from build123d import *

# Parameters (mm, degrees)
SKETCH1_R           = 22.225
SKETCH1_R_2         = 8.001
BOSS_EXTRUDE1_DEPTH = 31.75
SKETCH2_R           = 1.5875
SKETCH2_R_2         = 8.001
CUT_EXTRUDE1_DEPTH  = 9.921875
FILLET1_R           = 3.175
SKETCH3_R           = 1.5875
CUT_EXTRUDE2_DEPTH  = 45.676210112


with BuildPart() as part:
    # Sketch1 → Boss-Extrude1 (new body)
    with BuildSketch(Plane(origin=(0, 0, 0), x_dir=(1, 0, 0), z_dir=(0, 1, 0))):
        with Locations(Location((0, 0, 0), (0, 0, 270))):
            Circle(SKETCH1_R)
        with Locations(Location((0, 0, 0), (0, 0, 270))):
            Circle(SKETCH1_R_2, mode=Mode.SUBTRACT)
    extrude(amount=BOSS_EXTRUDE1_DEPTH)

    # Sketch2 → Cut-Extrude1 (cut)
    # profile 1 of 31: a face of its own
    with BuildSketch(Plane.XZ):
        with BuildLine():
            ThreePointArc((-12.2555, 0), (-12.468184671, 0.79375), (-13.04925, 1.374815329))
            Line((-13.04925, 1.374815329), (-13.843, 0))
            Line((-13.843, 0), (-13.04925, -1.374815329))
            ThreePointArc((-13.04925, -1.374815329), (-12.468184671, -0.79375), (-12.2555, 0))
        make_face()
    # profile 2 of 31: a face of its own
    with BuildSketch(Plane.XZ):
        with BuildLine():
            Line((-13.843, 0), (-13.04925, 1.374815329))
            ThreePointArc((-13.04925, 1.374815329), (-15.4305, 0), (-13.04925, -1.374815329))
            Line((-13.04925, -1.374815329), (-13.843, 0))
        make_face()
    # profile 3 of 31: a face of its own
    with BuildSketch(Plane.XZ):
        with BuildLine():
            ThreePointArc((-12.2555, 0), (-12.468184671, 0.79375), (-13.04925, 1.374815329))
            Line((-13.04925, 1.374815329), (-13.843, 0))
            Line((-13.843, 0), (-13.04925, -1.374815329))
            ThreePointArc((-13.04925, -1.374815329), (-12.468184671, -0.79375), (-12.2555, 0))
        make_face()
    # profile 4 of 31: a face of its own
    with BuildSketch(Plane.XZ):
        with BuildLine():
            Line((-13.843, 0), (-13.04925, 1.374815329))
            ThreePointArc((-13.04925, 1.374815329), (-15.4305, 0), (-13.04925, -1.374815329))
            Line((-13.04925, -1.374815329), (-13.843, 0))
        make_face()
    # profile 5 of 31: a face of its own
    with BuildSketch(Plane.XZ):
        with Locations((-13.843, 0)):
            Circle(SKETCH2_R)
    # profile 6 of 31: a face of its own
    with BuildSketch(Plane.XZ):
        with Locations((-6.9215, -11.988389665)):
            Circle(SKETCH2_R)
    # profile 7 of 31: a face of its own
    with BuildSketch(Plane.XZ):
        with Locations((6.9215, -11.988389665)):
            Circle(SKETCH2_R)
    # profile 8 of 31: a face of its own
    with BuildSketch(Plane.XZ):
        with Locations((13.843, 0)):
            Circle(SKETCH2_R)
    # profile 9 of 31: a face of its own
    with BuildSketch(Plane.XZ):
        with Locations((6.9215, 11.988389665)):
            Circle(SKETCH2_R)
    # profile 10 of 31: a face of its own
    with BuildSketch(Plane.XZ):
        with Locations((-6.9215, 11.988389665)):
            Circle(SKETCH2_R)
    # profile 11 of 31: a face of its own
    with BuildSketch(Plane.XZ):
        Polygon((-13.843, 0), (-6.9215, -11.988389665), (6.9215, -11.988389665), (13.843, 0), (6.9215, 11.988389665), (-6.9215, 11.988389665), align=None)
        with Locations(Location((0, 0, 0), (0, 0, 270))):
            Circle(SKETCH2_R_2, mode=Mode.SUBTRACT)
    # profile 12 of 31: a face of its own
    with BuildSketch(Plane.XZ):
        with BuildLine():
            ThreePointArc((-5.334, -11.988389665), (-6.12775, -10.613574336), (-7.71525, -10.613574336))
            Line((-7.71525, -10.613574336), (-6.9215, -11.988389665))
            Line((-6.9215, -11.988389665), (-5.334, -11.988389665))
        make_face()
    # profile 13 of 31: a face of its own
    with BuildSketch(Plane.XZ):
        with BuildLine():
            Line((-6.9215, -11.988389665), (-7.71525, -10.613574336))
            ThreePointArc((-7.71525, -10.613574336), (-7.71525, -13.363204993), (-5.334, -11.988389665))
            Line((-5.334, -11.988389665), (-6.9215, -11.988389665))
        make_face()
    # profile 14 of 31: a face of its own
    with BuildSketch(Plane.XZ):
        with BuildLine():
            ThreePointArc((-5.334, -11.988389665), (-6.12775, -10.613574336), (-7.71525, -10.613574336))
            Line((-7.71525, -10.613574336), (-6.9215, -11.988389665))
            Line((-6.9215, -11.988389665), (-5.334, -11.988389665))
        make_face()
    # profile 15 of 31: a face of its own
    with BuildSketch(Plane.XZ):
        with BuildLine():
            Line((-6.9215, -11.988389665), (-7.71525, -10.613574336))
            ThreePointArc((-7.71525, -10.613574336), (-7.71525, -13.363204993), (-5.334, -11.988389665))
            Line((-5.334, -11.988389665), (-6.9215, -11.988389665))
        make_face()
    # profile 16 of 31: a face of its own
    with BuildSketch(Plane.XZ):
        with BuildLine():
            ThreePointArc((8.509, -11.988389665), (8.296315329, -11.194639665), (7.71525, -10.613574336))
            Line((7.71525, -10.613574336), (6.9215, -11.988389665))
            Line((6.9215, -11.988389665), (5.334, -11.988389665))
            ThreePointArc((5.334, -11.988389665), (6.9215, -13.575889665), (8.509, -11.988389665))
        make_face()
    # profile 17 of 31: a face of its own
    with BuildSketch(Plane.XZ):
        with BuildLine():
            Line((6.9215, -11.988389665), (7.71525, -10.613574336))
            ThreePointArc((7.71525, -10.613574336), (6.12775, -10.613574336), (5.334, -11.988389665))
            Line((5.334, -11.988389665), (6.9215, -11.988389665))
        make_face()
    # profile 18 of 31: a face of its own
    with BuildSketch(Plane.XZ):
        with BuildLine():
            ThreePointArc((8.509, -11.988389665), (8.296315329, -11.194639665), (7.71525, -10.613574336))
            Line((7.71525, -10.613574336), (6.9215, -11.988389665))
            Line((6.9215, -11.988389665), (5.334, -11.988389665))
            ThreePointArc((5.334, -11.988389665), (6.9215, -13.575889665), (8.509, -11.988389665))
        make_face()
    # profile 19 of 31: a face of its own
    with BuildSketch(Plane.XZ):
        with BuildLine():
            Line((6.9215, -11.988389665), (7.71525, -10.613574336))
            ThreePointArc((7.71525, -10.613574336), (6.12775, -10.613574336), (5.334, -11.988389665))
            Line((5.334, -11.988389665), (6.9215, -11.988389665))
        make_face()
    # profile 20 of 31: a face of its own
    with BuildSketch(Plane.XZ):
        with BuildLine():
            ThreePointArc((15.4305, 0), (14.63675, 1.374815329), (13.04925, 1.374815329))
            Line((13.04925, 1.374815329), (13.843, 0))
            Line((13.843, 0), (13.04925, -1.374815329))
            ThreePointArc((13.04925, -1.374815329), (14.63675, -1.374815329), (15.4305, 0))
        make_face()
    # profile 21 of 31: a face of its own
    with BuildSketch(Plane.XZ):
        with BuildLine():
            Line((13.843, 0), (13.04925, 1.374815329))
            ThreePointArc((13.04925, 1.374815329), (12.2555, 0), (13.04925, -1.374815329))
            Line((13.04925, -1.374815329), (13.843, 0))
        make_face()
    # profile 22 of 31: a face of its own
    with BuildSketch(Plane.XZ):
        with BuildLine():
            ThreePointArc((15.4305, 0), (14.63675, 1.374815329), (13.04925, 1.374815329))
            Line((13.04925, 1.374815329), (13.843, 0))
            Line((13.843, 0), (13.04925, -1.374815329))
            ThreePointArc((13.04925, -1.374815329), (14.63675, -1.374815329), (15.4305, 0))
        make_face()
    # profile 23 of 31: a face of its own
    with BuildSketch(Plane.XZ):
        with BuildLine():
            Line((13.843, 0), (13.04925, 1.374815329))
            ThreePointArc((13.04925, 1.374815329), (12.2555, 0), (13.04925, -1.374815329))
            Line((13.04925, -1.374815329), (13.843, 0))
        make_face()
    # profile 24 of 31: a face of its own
    with BuildSketch(Plane.XZ):
        with BuildLine():
            ThreePointArc((8.509, 11.988389665), (6.9215, 13.575889665), (5.334, 11.988389665))
            Line((5.334, 11.988389665), (6.9215, 11.988389665))
            Line((6.9215, 11.988389665), (7.71525, 10.613574336))
            ThreePointArc((7.71525, 10.613574336), (8.296315329, 11.194639665), (8.509, 11.988389665))
        make_face()
    # profile 25 of 31: a face of its own
    with BuildSketch(Plane.XZ):
        with BuildLine():
            Line((6.9215, 11.988389665), (5.334, 11.988389665))
            ThreePointArc((5.334, 11.988389665), (6.12775, 10.613574336), (7.71525, 10.613574336))
            Line((7.71525, 10.613574336), (6.9215, 11.988389665))
        make_face()
    # profile 26 of 31: a face of its own
    with BuildSketch(Plane.XZ):
        with BuildLine():
            ThreePointArc((8.509, 11.988389665), (6.9215, 13.575889665), (5.334, 11.988389665))
            Line((5.334, 11.988389665), (6.9215, 11.988389665))
            Line((6.9215, 11.988389665), (7.71525, 10.613574336))
            ThreePointArc((7.71525, 10.613574336), (8.296315329, 11.194639665), (8.509, 11.988389665))
        make_face()
    # profile 27 of 31: a face of its own
    with BuildSketch(Plane.XZ):
        with BuildLine():
            Line((6.9215, 11.988389665), (5.334, 11.988389665))
            ThreePointArc((5.334, 11.988389665), (6.12775, 10.613574336), (7.71525, 10.613574336))
            Line((7.71525, 10.613574336), (6.9215, 11.988389665))
        make_face()
    # profile 28 of 31: a face of its own
    with BuildSketch(Plane.XZ):
        with BuildLine():
            ThreePointArc((-7.71525, 10.613574336), (-6.12775, 10.613574336), (-5.334, 11.988389665))
            Line((-5.334, 11.988389665), (-6.9215, 11.988389665))
            Line((-6.9215, 11.988389665), (-7.71525, 10.613574336))
        make_face()
    # profile 29 of 31: a face of its own
    with BuildSketch(Plane.XZ):
        with BuildLine():
            Line((-6.9215, 11.988389665), (-5.334, 11.988389665))
            ThreePointArc((-5.334, 11.988389665), (-7.71525, 13.363204993), (-7.71525, 10.613574336))
            Line((-7.71525, 10.613574336), (-6.9215, 11.988389665))
        make_face()
    # profile 30 of 31: a face of its own
    with BuildSketch(Plane.XZ):
        with BuildLine():
            ThreePointArc((-7.71525, 10.613574336), (-6.12775, 10.613574336), (-5.334, 11.988389665))
            Line((-5.334, 11.988389665), (-6.9215, 11.988389665))
            Line((-6.9215, 11.988389665), (-7.71525, 10.613574336))
        make_face()
    # profile 31 of 31: a face of its own
    with BuildSketch(Plane.XZ):
        with BuildLine():
            Line((-6.9215, 11.988389665), (-5.334, 11.988389665))
            ThreePointArc((-5.334, 11.988389665), (-7.71525, 13.363204993), (-7.71525, 10.613574336))
            Line((-7.71525, 10.613574336), (-6.9215, 11.988389665))
        make_face()
    extrude(amount=-CUT_EXTRUDE1_DEPTH, mode=Mode.SUBTRACT)

    # Fillet1
    fillet1_edges = [part.edges().sort_by_distance(p)[0] for p in [
        (-5.334, 4.9609375, -11.988389665),
        (-7.71525, 4.9609375, -10.613574336),
        (-13.04925, 4.9609375, -1.374815329),
        (-13.04925, 4.9609375, 1.374815329),
        (-7.71525, 4.9609375, 10.613574336),
        (-5.334, 4.9609375, 11.988389665),
        (5.334, 4.9609375, 11.988389665),
        (7.71525, 4.9609375, 10.613574336),
        (13.04925, 4.9609375, 1.374815329),
        (13.04925, 4.9609375, -1.374815329),
        (7.71525, 4.9609375, -10.613574336),
        (5.334, 4.9609375, -11.988389665),
    ]]
    fillet(fillet1_edges, radius=FILLET1_R)

    # Sketch3 → Cut-Extrude2 (cut, through all)
    with BuildSketch(Plane.XZ):
        with Locations(Location((0, 16.51, 0), (0, 0, 270))):
            Circle(SKETCH3_R)
        with Locations(Location((14.298079416, -8.255, 0), (0, 0, 270))):
            Circle(SKETCH3_R)
        with Locations(Location((-14.298079416, -8.255, 0), (0, 0, 270))):
            Circle(SKETCH3_R)
    extrude(amount=-CUT_EXTRUDE2_DEPTH, mode=Mode.SUBTRACT)


solid = part.part
Read the model definition and answer for the solid it produces. Units are mm, in the model's axes. A direction names the side the tool comes from. Coordinates: 2 decimals unless noted, no trailing zeros. Loops run counter-clockwise (first coordinate to the right, second up) from the corner with the lowest first, then second, coordinate; pieces in that order, holes last.
Q1. Consider probe 1 along X at (y, z) = (22, 0) (3 decimals); probe 2 along Y at (x, z) = (-11, 0.5); probe 3 along X at (y, z) = (30.5, -18). Determine where each line is inside the solid, lowest interval first.
Q2. The part is cut by section A-A on x = 0. Give the number of separate pieces and of enclosed holes in the cut face, and give its area (3 significant figures).
Q3. The mould has two halves that part along Z. Classify faces 3 (the face through (-8.286, 5.03, 10.194)), 4 (the face through (-8.286, 5.03, -10.194)), 5 (the face through (-10, 0, 10)): +Z half, -Z half, draft (parallel to the pull), parting line (faces both ways), or undercut.
Q4. Which of the six approach directions +Z, -Z, +X, -X, +Y, -Y give full straight-line access (tool end or side, diameter ignored) to faces 1 (the face through (0.477, 15.653, 14.996)), 2 (the face through (-7.74, 4.89, -13.35))?
Q5. Each of these flat-tipped pins is pushed along its axis until it touches: pin 1 Ø8 at (x, z) = (-5.5, 2.5) entering from -Y; pin 2 Ø3 at (x, y) = (-15.5, 25) entering from -Z; pin 3 Ø9.5 at (x, z) = (0, 0) entering from -Y; pin 4 Ø12 at (y, z) = (13, -15) entering from -X. Where does it stop, or does it pass through?
Q6. The part is cut by section C-C on x = 5. Write down the section's boundary in (y, z), and give its area (3 significant figures).
Results below:
1. probe 1: x = -22.225 to -8.001, 8.001 to 22.225
1. probe 2: y = 9.92 to 31.75
1. probe 3: x = -13.04 to 13.04
2. separate pieces: 3
2. enclosed holes: 0
2. area: 723 mm2
3. face 3: undercut
3. face 4: undercut
3. face 5: draft
4. face 1: +Y, -Y
4. face 2: -Y
5. pin 1: stops at y = 9.92
5. pin 2: stops at z = -17.26
5. pin 3: passes through
5. pin 4: stops at x = -20.32
6. outline: (0, -21.66) - (31.75, -21.66) - (31.75, -6.25) - (9.92, -6.25) - (9.92, -12.44) - (0, -12.44) - close; (0, 12.44) - (9.92, 12.44) - (9.92, 6.25) - (31.75, 6.25) - (31.75, 21.66) - (0, 21.66) - close
6. area: 856 mm2
